Geometry check sheet. Reference: drawing and pictorial views, mm from the part's lowest x, y, z. A direction names the side the tool comes from. Coordinates: 2 decimals unless noted, no trailing zeros. Write each loop counter-clockwise with the first axis right and the second up, starting at its lowest first coordinate (ties: lowest second). Pieces come first, ordered by that corner, then holes. Notation, with made-up numbers: (15.5, -0.5) -> (43.5, -0.5) arc R21 ccw to (43.5, 12.5) -> close; hole circle Ø3 at (75, 8.5). An arc over 180 degrees is marked (long way). Put each result on its own line as item: value.
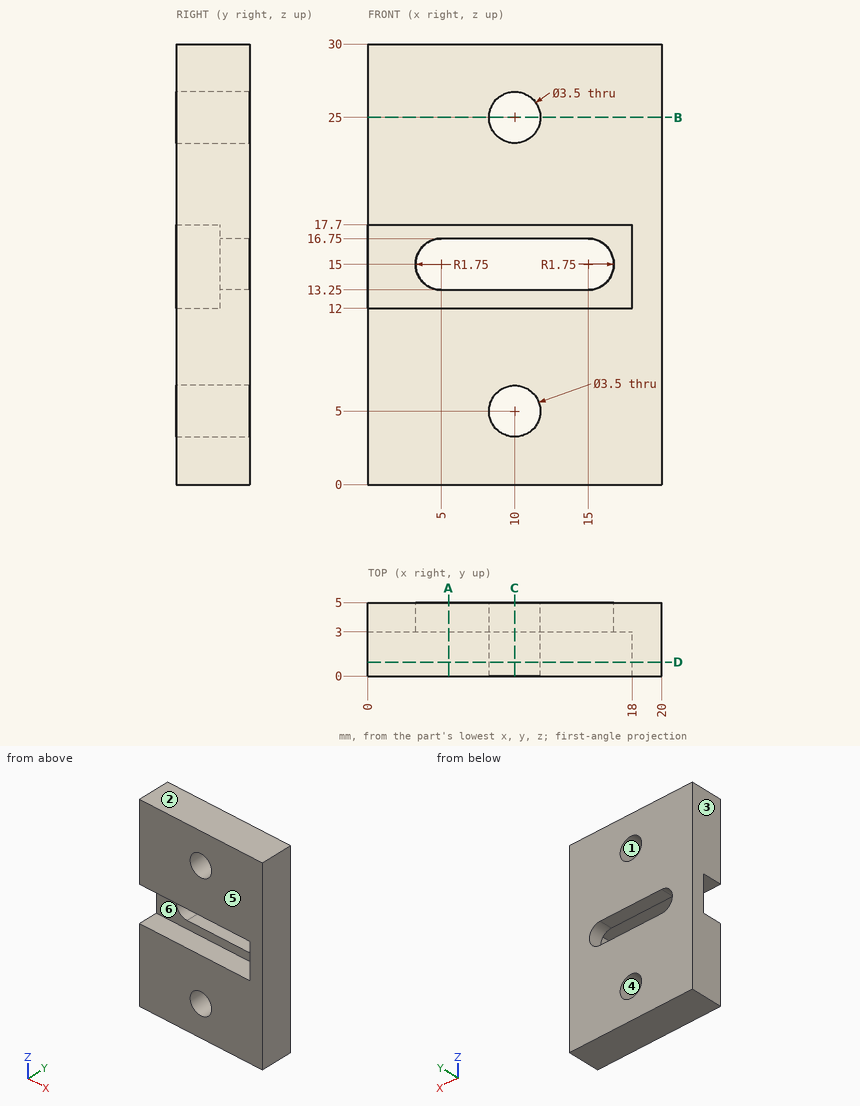
Q1. Cross-section at D-D (y = 0.95). Record the cut outline in (x, z).
Recorded:
outline: (0, 0) -> (20, 0) -> (20, 30) -> (0, 30) -> (0, 17.7) -> (18, 17.7) -> (18, 12) -> (0, 12) -> close; hole circle Ø3.5 at (10, 5); hole circle Ø3.5 at (10, 25)
Q2. Cross-section at A-A (x = 5.5). Record the cut outline in (y, z).
Recorded:
outline: (0, 0) -> (5, 0) -> (5, 13.25) -> (3, 13.25) -> (3, 12) -> (0, 12) -> close; (0, 17.7) -> (3, 17.7) -> (3, 16.75) -> (5, 16.75) -> (5, 30) -> (0, 30) -> close
Q3. Cross-section at B-B (z = 25). Record the cut outline in (x, y), plus the area to 3 significant figures.
Recorded:
outline: (0, 0) -> (8.25, 0) -> (8.25, 5) -> (0, 5) -> close; (11.75, 0) -> (20, 0) -> (20, 5) -> (11.75, 5) -> close
area: 82.5 mm2
Q4. Tool access check on the marked faces 5 and 6. Record the directions out of +Z, -Z, +X, -X, +Y, -Y that give a thin tool (end or side, any length) a straight path to the whole face; none if there is none.
Recorded:
face 5: +Z, -Z, +X, -X, -Y
face 6: -X, -Y
Q5. Depth check by flat-ended pin: P1, Ø3, axis at x = 12, z = 14, coming from the -Y side; P2, Ø0.9, axis at y = 1, z = 16, coming from the -X side. Enter the tip coordinate at first touch or a pass-through.
Recorded:
P1: stops at y = 3
P2: stops at x = 18
Q6. Material ranges on line 1 along Z through (x, y) = (7, 3.1); line 2 along X through (y, z) = (1.55, 25); line 3 along Z through (x, y) = (11.25, 4), recorded low to high.
Recorded:
line 1: z = 0 to 13.25, 16.75 to 30
line 2: x = 0 to 8.25, 11.75 to 20
line 3: z = 0 to 3.78, 6.22 to 13.25, 16.75 to 23.78, 26.22 to 30
Q7. Cross-section at C-C (x = 10). Record the cut outline in (y, z).
Recorded:
outline: (0, 0) -> (5, 0) -> (5, 3.25) -> (0, 3.25) -> close; (0, 6.75) -> (5, 6.75) -> (5, 13.25) -> (3, 13.25) -> (3, 12) -> (0, 12) -> close; (0, 17.7) -> (3, 17.7) -> (3, 16.75) -> (5, 16.75) -> (5, 23.25) -> (0, 23.25) -> close; (0, 26.75) -> (5, 26.75) -> (5, 30) -> (0, 30) -> close
Q8. Mould release check, pull along X, two halves, no side actions. Record for the marked faces 1, 2, 3 and 4: released by +X, released by -X, zero draft, split by the parting line, or undercut.
Recorded:
face 1: undercut
face 2: zero draft
face 3: released by -X
face 4: undercut
